Work out the finished part from the listing and answer in its coordinate system (mm). A direction names the side the tool comes from. Coordinates: 2 decimals unless noted, no trailing zeros. Order: outer loops, then holes, each group sorted by start corner. A loop starts at its lowest first (then second) coordinate and runs counter-clockwise, first axis right, second up. Notation, with made-up numbers: M 78,52 L 134,52 A22 ccw 134,74 Z; hole C 34.25,29 d2. An arc over 180 degrees is marked long. Use a Markdown table: item, result.
from build123d import *

# Parameters (mm, degrees)
BOSS_EXTRUDE1_START = -10
BOSS_EXTRUDE1_DEPTH = 35
CHAMFER1_SIZE       = 0.5


with BuildPart() as part:
    # Sketch1 → Boss-Extrude1 (new body)
    with BuildSketch(Plane(origin=(0, 0, 0), x_dir=(0, 0, -1), z_dir=(1, 0, 0)).offset(BOSS_EXTRUDE1_START)):
        Polygon((-8.0829, 0), (-4.04145, -6.999996736), (4.04145, -6.999996736), (8.0829, 0), (4.04145, 6.999996736), (-4.04145, 6.999996736), align=None)
    extrude(amount=BOSS_EXTRUDE1_DEPTH)

    # Sketch2 → Cut-Revolve1 (revolve, cut)
    with BuildSketch(Plane(origin=(0, 0, 0), x_dir=(1, 0, 0), z_dir=(0, 1, 0)), mode=Mode.PRIVATE) as cut_revolve1_sk:
        Polygon((0, 8.0829), (-10, 8.0829), (-10, 4), (-1, 4), (-1, 3.45), (0, 3.45), align=None)
    revolve(cut_revolve1_sk.sketch.rotate(Axis((-12.627683811, 0, 0), (1, 0, 0)), 180), axis=Axis((-12.627683811, 0, 0), (1, 0, 0)), mode=Mode.SUBTRACT)

    # Sketch3 → Cut-Revolve2 (revolve, cut)
    with BuildSketch(Plane(origin=(0, 0, 0), x_dir=(1, 0, 0), z_dir=(0, 1, 0)), mode=Mode.PRIVATE) as cut_revolve2_sk:
        Polygon((25, 8.0829), (25, 3), (17, 3), (17, 4), (5.9, 4), (5.9, 5), (4.9, 5), (4.9, 8.0829), align=None)
    revolve(cut_revolve2_sk.sketch.rotate(Axis((-14.24617289, 0, 0), (1, 0, 0)), 180), axis=Axis((-14.24617289, 0, 0), (1, 0, 0)), mode=Mode.SUBTRACT)

    # Chamfer1
    chamfer1_edges = [part.edges().sort_by_distance(p)[0] for p in [
        (-10, 0, -4),
        (25, 0, -3),
    ]]
    chamfer(chamfer1_edges, length=CHAMFER1_SIZE)


solid = part.part
1. Section D-D on z = -5.5 is taken. Determine the outline of the cut face in (x, y), then the cut area to 3 significant figures.
Answers below:
| item | result |
|---|---|
| outline | M 0,-4.47 L 4.9,-4.47 L 4.9,4.47 L 0,4.47 Z |
| area | 43.8 mm² |
2. Find the intervals of material crossed by probe 1 along X at (y, z) = (3, -2.75); probe 2 along X at (y, z) = (6.25, 1); probe 3 along Y at (x, z) = (18, 0), in increasing order.
Answers below:
| item | result |
|---|---|
| probe 1 | 0 to 5.9 |
| probe 2 | 0 to 4.9 |
| probe 3 | -3 to 3 |
3. Section B-B on x = 3 is taken. Determine the outline of the cut face in (y, z), then the cut area to 3 significant figures.
Answers below:
| item | result |
|---|---|
| outline | M -7,-4.04 L 0,-8.08 L 7,-4.04 L 7,4.04 L 0,8.08 L -7,4.04 Z |
| area | 170 mm² |
4. Section C-C on x = 22.5 is taken. Determine the outline of the cut face in (y, z).
Answers below:
| item | result |
|---|---|
| outline | C 0,0 d6 |
5. Flat-ended cylindrical pins translate along their axes: P1, Ø8, axis at x = -6.5, y = -1, coming from the +Z side; P2, Ø1, axis at y = 2.5, z = -5.5, coming from the +X side; P3, Ø2, axis at x = 19, y = -1.5, coming from the +Z side. Find the tip coordinate at first contact, or state that the pin passes through.
Answers below:
| item | result |
|---|---|
| P1 | z = 4 |
| P2 | x = 4.9 |
| P3 | z = 2.96 |
6. Section A-A on z = 0 is taken. Determine the outline of the cut face in (x, y).
Answers below:
| item | result |
|---|---|
| outline | M -10,-3.5 L -9.5,-4 L -1,-4 L -1,-3.45 L 0,-3.45 L 0,-7 L 4.9,-7 L 4.9,-5 L 5.9,-5 L 5.9,-4 L 17,-4 L 17,-3 L 24.5,-3 L 25,-2.5 L 25,2.5 L 24.5,3 L 17,3 L 17,4 L 5.9,4 L 5.9,5 L 4.9,5 L 4.9,7 L 0,7 L 0,3.45 L -1,3.45 L -1,4 L -9.5,4 L -10,3.5 Z |
7. For a pull along X with two mould halves and no side action, classify faces 1 (the face through (-0.493, -2.332, -2.543)), 2 (the face through (17, -3, -1)), 3 (the face through (-5.19, 3.905, -0.867)) as +X half, -X half, draft (parallel to the pull), parting line (faces both ways), or undercut.
Answers below:
| item | result |
|---|---|
| face 1 | undercut |
| face 2 | +X half |
| face 3 | draft |
8. For faces 4 (the face through (11.372, 3.905, -0.867)), 5 (the face through (2, 7, 0)), determine the directions among +Z, -Z, +X, -X, +Y, -Y from which every point of the face is accessible in a straight line to the end or side of a thin tool.
Answers below:
| item | result |
|---|---|
| face 4 | +X |
| face 5 | +Z, -Z, +X, -X, +Y |
